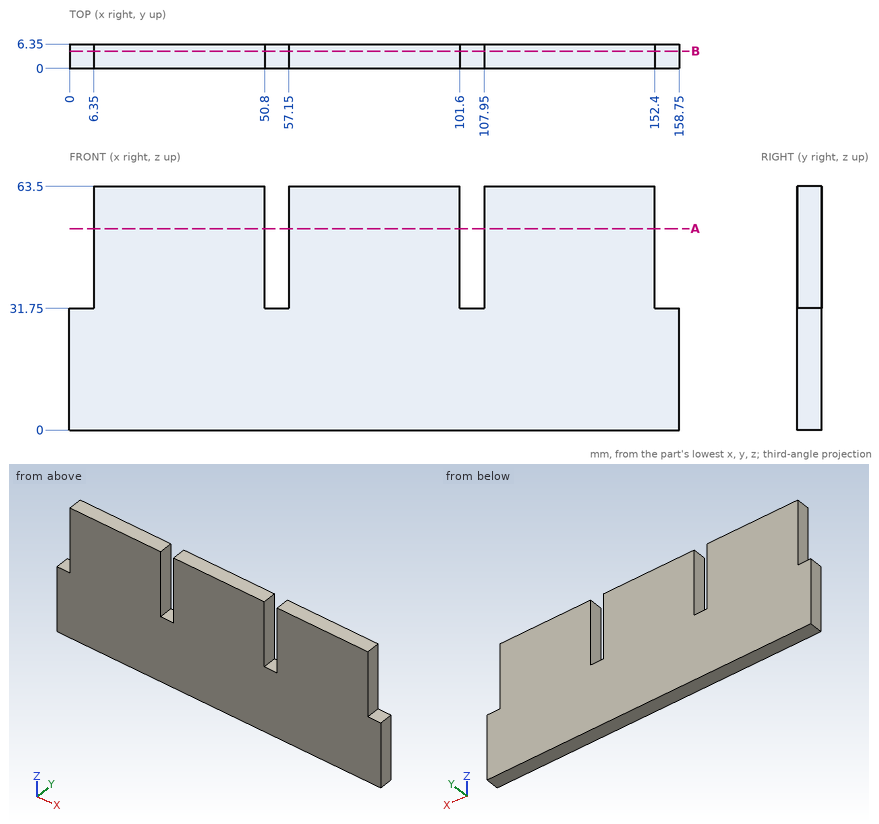
Part print with two shaded views. Sizes in mm from the minimum x, y, z corner. Round coordinates to 2 decimals unless told otherwise and drop trailing zeros. Loops run counter-clockwise (first coordinate to the right, second up) from the corner with the lowest first, then second, coordinate; pieces in that order, holes last. Notation, with made-up numbers: (8.5, 72) - (65.5, 72) arc R11 cw to (65.5, 77) - close; hole circle Ø4 at (43.25, 26). An arc over 180 degrees is marked (long way). Put each result on its own line as item: value.
1. Slice it at A-A on z = 52.5. List the corners of the cut face in (x, y), and give its area (3 significant figures).
Geometry check:
outline: (6.35, 0) - (50.8, 0) - (50.8, 6.35) - (6.35, 6.35) - close; (57.15, 0) - (101.6, 0) - (101.6, 6.35) - (57.15, 6.35) - close; (107.95, 0) - (152.4, 0) - (152.4, 6.35) - (107.95, 6.35) - close
area: 847 mm²
2. Pin check, flat tips, straight feed: P1, Ø3, axis at x = 154, y = 3, coming from the +Z side; P2, Ø1.9, axis at y = 4, z = 44.5, coming from the +X side; P3, Ø3, axis at y = 4, z = 40.5, coming from the -X side. Stop position of each tip, or through.
Geometry check:
P1: z = 31.75
P2: x = 152.4
P3: x = 6.35
3. Slice it at B-B on y = 4.5. List the corners of the cut face in (x, z), and give its area (3 significant figures).
Geometry check:
outline: (0, 0) - (158.75, 0) - (158.75, 31.75) - (152.4, 31.75) - (152.4, 63.5) - (107.95, 63.5) - (107.95, 31.75) - (101.6, 31.75) - (101.6, 63.5) - (57.15, 63.5) - (57.15, 31.75) - (50.8, 31.75) - (50.8, 63.5) - (6.35, 63.5) - (6.35, 31.75) - (0, 31.75) - close
area: 9,270 mm²
4. Wall check: line 1 (X direction, y = 3.75, z = 34.5); line 2 (Z direction, x = 52.5, y = 2). Give the ranges that are in metal, low to high.
Geometry check:
line 1: 6.35 to 50.8, 57.15 to 101.6, 107.95 to 152.4
line 2: 0 to 31.75
